Model file for the job. Use its own axes, mm. Face numbers are marked on the shaded views. Give positions to 0.01 mm unless a question says otherwise; leave off trailing zeros. Order: outer loops, then holes, each group sorted by start corner. A loop starts at its lowest first (then second) coordinate and runs counter-clockwise, first axis right, second up. Notation, with made-up numbers: M -2.5,72.5 L 2.5,72.5 A11 cw 2.5,76.5 Z; hole C 66,86 d2. An arc over 180 degrees is marked long. Return JSON: item names as keys, results as strings. Group by question number.
1. Pin check, flat tip, straight feed: pin 1 (2 mm diameter, centred on x = 141.5, y = 52.5, fed in from -Z). Stop position of the tip, or through.
2. Slice it at A-A on z = 16. List the corners of the cut face in (x, y) (3 decimals), then the cut area to 3 significant figures.
3. Wall check: probe 1 along X at (y, z) = (66.5, 2) (3 decimals); probe 2 along Z at (x, y) = (108.5, 65.5); probe 3 along X at (y, z) = (17, 24.5). Give the ranges that are in metal, low to high. Write a range as [from, to].
4. Two-plate mould, pull along X, no slides. Class the marked faces 1, 2, 3 and 4: released by +X, released by -X, zero draft, split by the parting line, or undercut.
5. Slice it at B-B on y = 101. List the corners of the cut face in (x, z) (3 decimals), then the cut area to 3 significant figures.
6. Slice it at C-C on x = 95. List the corners of the cut face in (y, z).
from build123d import *

# Parameters (mm, degrees)
F1_DEPTH = 124.46
F3_D     = 4.4958


with BuildPart() as f1:
    # F0 (on Front) → F1 (new body)
    with BuildSketch(Plane.XZ):
        with BuildLine():
            Line((0, 21.3614), (0, 0))
            Line((0, 0), (2.0574, 0))
            Line((2.0574, 0), (2.0574, 21.3614))
            ThreePointArc((2.0574, 21.3614), (3.456024, 24.737976), (6.8326, 26.1366))
            Line((6.8326, 26.1366), (174.1424, 26.1366))
            ThreePointArc((174.1424, 26.1366), (177.518976, 24.737976), (178.9176, 21.3614))
            Line((178.9176, 21.3614), (178.9176, 0))
            Line((178.9176, 0), (180.975, 0))
            Line((180.975, 0), (180.975, 21.3614))
            ThreePointArc((180.975, 21.3614), (178.973778, 26.192778), (174.1424, 28.194))
            Line((174.1424, 28.194), (6.8326, 28.194))
            ThreePointArc((6.8326, 28.194), (2.001222, 26.192778), (0, 21.3614))
        make_face()
    extrude(amount=-F1_DEPTH)

    # F3 (through all)
    with Locations(Plane.YZ.offset(180.975)):
        with Locations((19.3675, 7.9502), (105.0925, 7.9502)):
            Hole(F3_D / 2)


solid = f1.part
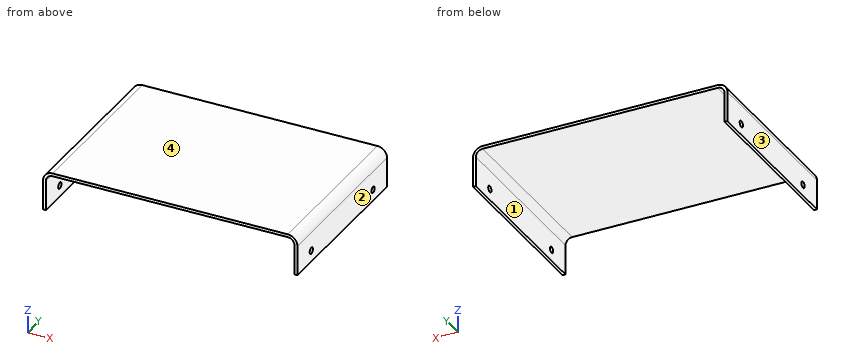
Result:
{
 "1": {"pin 1": "stops at z = 26.14"},
 "2": {"outline": "M 0,0 L 2.057,0 L 2.057,124.46 L 0,124.46 Z; M 178.918,0 L 180.975,0 L 180.975,124.46 L 178.918,124.46 Z", "area": "512 mm2"},
 "3": {"probe 1": "x = [0, 2.057], [178.918, 180.975]", "probe 2": "z = [26.14, 28.19]", "probe 3": "x = [0.76, 3.23], [177.74, 180.21]"},
 "4": {"face 1": "undercut", "face 2": "released by +X", "face 3": "released by -X", "face 4": "zero draft"},
 "5": {"outline": "M 0,0 L 2.057,0 L 2.057,21.361 A4.775 cw 6.833,26.137 L 174.142,26.137 A4.775 cw 178.918,21.361 L 178.918,0 L 180.975,0 L 180.975,21.361 A6.833 ccw 174.142,28.194 L 6.833,28.194 A6.833 ccw 0,21.361 Z", "area": "470 mm2"},
 "6": {"outline": "M 0,26.14 L 124.46,26.14 L 124.46,28.19 L 0,28.19 Z"}
}
